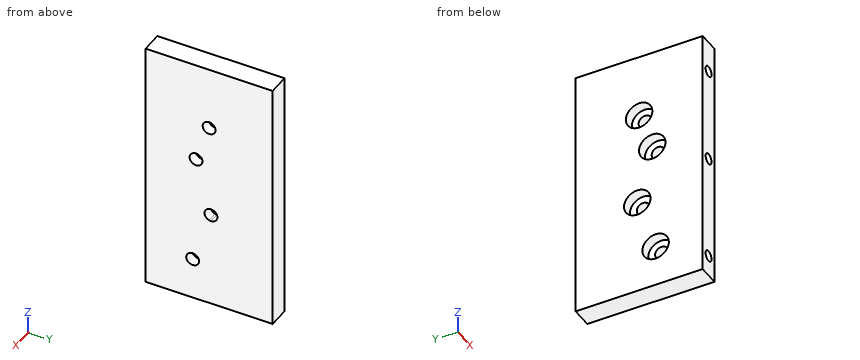
```python
from build123d import *

# Parameters (mm, degrees)
SKETCH1_R                       = 3.854557775
BOSS_EXTRUDE1_DEPTH             = 12.7
F_1_4_0_25_DIAMETER_HOLE2_D     = 6.35
F_1_4_0_25_DIAMETER_HOLE2_DEPTH = 12.7
F_1_4_0_25_DIAMETER_HOLE2_TIP   = 1.907732465
SKETCH2_R                       = 7.9375
CUT_EXTRUDE1_DEPTH              = 6.35


with BuildPart() as part:
    # Sketch1 → Boss-Extrude1 (new body)
    # profile 1 of 2: a face of its own
    with BuildSketch(Plane(origin=(0, 0, 0), x_dir=(0, 0, -1), z_dir=(1, 0, 0))):
        with BuildLine():
            Line((-76.2, 38.1), (-76.2, 0))
            Line((-76.2, 0), (-41.954557775, 0))
            ThreePointArc((-41.954557775, 0), (-38.1, 3.854557775), (-34.245442225, 0))
            Line((-34.245442225, 0), (14.762299925, 0))
            ThreePointArc((14.762299925, 0), (17.903949731, 4.910646748), (22.312291357, 1.096077429))
            ThreePointArc((22.312291357, 1.096077429), (22.272302901, 0.542293578), (22.153167239, 0))
            Line((22.153167239, 0), (76.2, 0))
            Line((76.2, 0), (76.2, 38.1))
            Line((76.2, 38.1), (-76.2, 38.1))
        make_face()
    # profile 2 of 2: a face of its own
    with BuildSketch(Plane(origin=(0, 0, 0), x_dir=(0, 0, -1), z_dir=(1, 0, 0))):
        with BuildLine():
            Line((-41.954557775, 0), (-76.2, 0))
            Line((-76.2, 0), (-76.2, -38.1))
            Line((-76.2, -38.1), (76.2, -38.1))
            Line((76.2, -38.1), (76.2, 0))
            Line((76.2, 0), (22.153167239, 0))
            ThreePointArc((22.153167239, 0), (18.457733582, -2.758480346), (14.762299925, 0))
            Line((14.762299925, 0), (-34.245442225, 0))
            ThreePointArc((-34.245442225, 0), (-38.1, -3.854557775), (-41.954557775, 0))
        make_face()
        with Locations((-14.836022013, -7.860160654)):
            Circle(SKETCH1_R, mode=Mode.SUBTRACT)
        with Locations((51.143457994, -9.873506971)):
            Circle(SKETCH1_R, mode=Mode.SUBTRACT)
    extrude(amount=BOSS_EXTRUDE1_DEPTH)

    # 1_4 _0.25_ Diameter Hole2
    with Locations(Plane.XZ.offset(38.1)):
        with Locations((6.35, 57.15), (6.35, -63.5), (6.35, 0)):
            Hole(F_1_4_0_25_DIAMETER_HOLE2_D / 2, depth=F_1_4_0_25_DIAMETER_HOLE2_DEPTH)
            with Locations((0, 0, -(F_1_4_0_25_DIAMETER_HOLE2_DEPTH + F_1_4_0_25_DIAMETER_HOLE2_TIP / 2))):  # 118° drill point
                Cone(0, F_1_4_0_25_DIAMETER_HOLE2_D / 2, F_1_4_0_25_DIAMETER_HOLE2_TIP, mode=Mode.SUBTRACT)

    # Sketch2 → Cut-Extrude1 (cut)
    with BuildSketch(Plane.ZY):
        with Locations((38.1, 0)):
            Circle(SKETCH2_R)
        with Locations((14.836022013, -7.860160654)):
            Circle(SKETCH2_R)
        with Locations((-18.457733582, 1.096077429)):
            Circle(SKETCH2_R)
        with Locations((-51.143457994, -9.873506971)):
            Circle(SKETCH2_R)
    extrude(amount=-CUT_EXTRUDE1_DEPTH, mode=Mode.SUBTRACT)


solid = part.part
```
Can you work these out from the model? Positions are in its coordinate system, mm. Give positions to 0.01 mm unless a question says otherwise; leave off trailing zeros. Loops run counter-clockwise (first coordinate to the right, second up) from the corner with the lowest first, then second, coordinate; pieces in that order, holes last. Notation, with made-up numbers: M 56,-11 L 86,-11 A28 ccw 86,15 Z; hole C -32,59.5 d8. An arc over 180 degrees is marked long. One line per item, written item: value.
(1) Suppose I cut it at B-B on y = -32. List the corners of the cut face in (x, z) for me (3 decimals), plus the area to 3 significant figures.
Returned:
outline: M 0,-76.2 L 12.7,-76.2 L 12.7,76.2 L 0,76.2 Z; hole C 6.35,-63.5 d6.35; hole C 6.35,0 d6.35; hole C 6.35,57.15 d6.35
area: 1,840 mm^2
(2) Will these pins go through, and if not, where does the flat tip stop? pin 1 (10 mm diameter, centred on y = 0, z = 38.1, fed in from -X); pin 2 (5 mm diameter, centred on x = 6.35, z = 57.15, fed in from -Y).
Returned:
pin 1: x = 6.35
pin 2: y = -24.99
(3) Suppose I cut it at C-C on x = 1.75. List the corners of the cut face in (y, z) for me (1 decimal).
Returned:
outline: M -38.1,-76.2 L 38.1,-76.2 L 38.1,76.2 L -38.1,76.2 Z; hole C -9.9,-51.1 d15.9; hole C -7.9,14.8 d15.9; hole C 0,38.1 d15.9; hole C 1.1,-18.5 d15.9
(4) Suppose I cut it at A-A on z = 38.1. List the corners of the cut face in (x, y) for me.
Returned:
outline: M 0,-38.1 L 12.7,-38.1 L 12.7,-3.85 L 6.35,-3.85 L 6.35,-7.94 L 0,-7.94 Z; M 0,7.94 L 6.35,7.94 L 6.35,3.85 L 12.7,3.85 L 12.7,38.1 L 0,38.1 Z
(5) Suppose I cut it at D-D on z = 14. List the corners of the cut face in (x, y) for me, plus the area to 3 significant figures.
Returned:
outline: M 0,-38.1 L 12.7,-38.1 L 12.7,-11.62 L 6.35,-11.62 L 6.35,-15.75 L 0,-15.75 Z; M 0,0.03 L 6.35,0.03 L 6.35,-4.1 L 12.7,-4.1 L 12.7,38.1 L 0,38.1 Z
area: 820 mm^2
(6) I need wall thicknesses on line 1 (Z direction, x = 8.5, y = 0); line 2 (Z direction, x = 6.35, y = -35.5) (3 decimals); line 3 (Z direction, x = 3.75, y = -6). Which ranges of each line are inside material? Lowest first, please.
Returned:
line 1: -76.2 to -22.15, -14.76 to 34.25, 41.95 to 76.2
line 2: -76.2 to -66.675, -60.325 to -3.175, 3.175 to 53.975, 60.325 to 76.2
line 3: -76.2 to -58.07, -44.22 to -22.01, -14.9 to 7.12, 22.55 to 32.9, 43.3 to 76.2
